Verification items for this drawing (mm, ordinates from the low corner). A direction names the side the tool comes from. Round coordinates to 2 decimals unless told otherwise and drop trailing zeros. Loops run counter-clockwise (first coordinate to the right, second up) from the corner with the lowest first, then second, coordinate; pieces in that order, holes last. Notation, with made-up numbers: M 5.5,-35.75 L 61.5,-35.75 A21 ccw 61.5,0.25 Z; hole C 11,24.25 d4. An arc over 180 degrees is marked long. One line per item, written item: value.
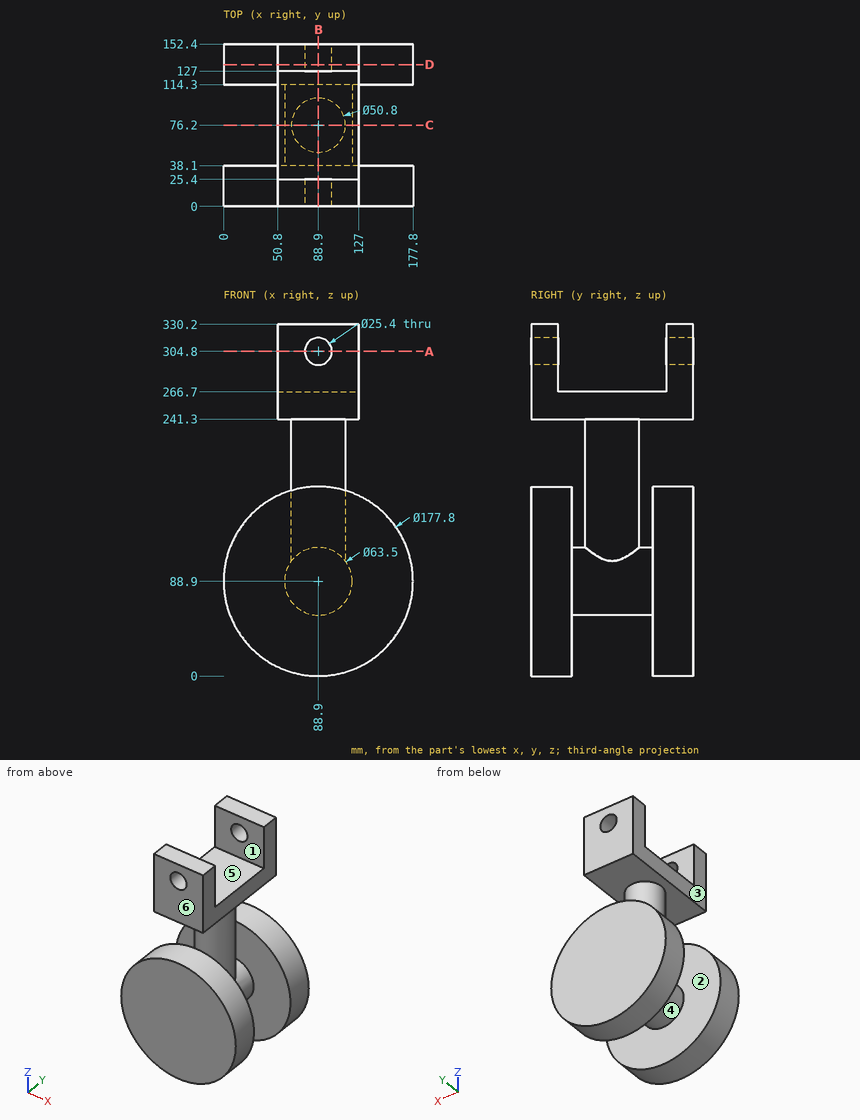
(1) Depth check by flat-ended pin: pin 1 Ø20.5 at (x, z) = (88.9, 304.8) entering from -Y; pin 2 Ø2 at (x, y) = (36.5, 135.5) entering from -Z; pin 3 Ø2 at (y, z) = (61.5, 112) entering from +X; pin 4 Ø1 at (x, z) = (101, 201) entering from +Y. Enter the tip coordinate at first touch or a pass-through.
Completed:
pin 1: passes through
pin 2: stops at z = 16.37
pin 3: stops at x = 111.7
pin 4: stops at y = 98.8
(2) Mould release check, pull along Z, two halves, no side actions. Record for the marked faces 4, 5 and 6: +Z half, -Z half, draft (parallel to the pull), parting line (faces both ways), or undercut.
Completed:
face 4: undercut
face 5: +Z half
face 6: draft
(3) Thickness scan on L1, parallel to Z at x = 88.9, y = 146; L2, parallel to Y at x = 90, z = 141; L3, parallel to Y at x = 62, z = 307.5. Record the ranges inside material, lowest first. Write a range as from..to.
Completed:
L1: z = 0..177.8, 241.3..292.1, 317.5..330.2
L2: y = 0..38.1, 50.82..101.58, 114.3..152.4
L3: y = 0..25.4, 127..152.4
(4) Sectioned sample at C-C on y = 76.2. Enter the section's corners in (x, z).
Completed:
outline: M 50.8,241.3 L 63.5,241.3 L 63.5,107.95 A31.75 ccw long 114.3,107.95 L 114.3,241.3 L 127,241.3 L 127,266.7 L 50.8,266.7 Z
(5) Sectioned sample at A-A on z = 304.8. Enter the section's corners in (x, y).
Completed:
outline: M 50.8,0 L 76.2,0 L 76.2,25.4 L 50.8,25.4 Z; M 50.8,127 L 76.2,127 L 76.2,152.4 L 50.8,152.4 Z; M 101.6,0 L 127,0 L 127,25.4 L 101.6,25.4 Z; M 101.6,127 L 127,127 L 127,152.4 L 101.6,152.4 Z
(6) Sectioned sample at B-B on x = 88.9. Count the separate pieces of the cut face and the enclosed holes in it, and give its area (3 significant figures).
Completed:
separate pieces: 3
enclosed holes: 0
area: 30,300 mm^2
(7) Tool access check on the marked faces 1, 2 and 3. Record the directions out of +Z, -Z, +X, -X, +Y, -Y that give a thin tool (end or side, any length) a straight path to the whole face; none if there is none.
Completed:
face 1: +Z, +X, -X
face 2: none
face 3: +Z, -X, +Y, -Y
(8) Sectioned sample at D-D on y = 133. Enter the section's corners in (x, z), and give its area (3 significant figures).
Completed:
outline: C 88.9,88.9 d177.8; M 50.8,241.3 L 127,241.3 L 127,330.2 L 50.8,330.2 Z; hole C 88.9,304.8 d25.4
area: 31,100 mm^2
